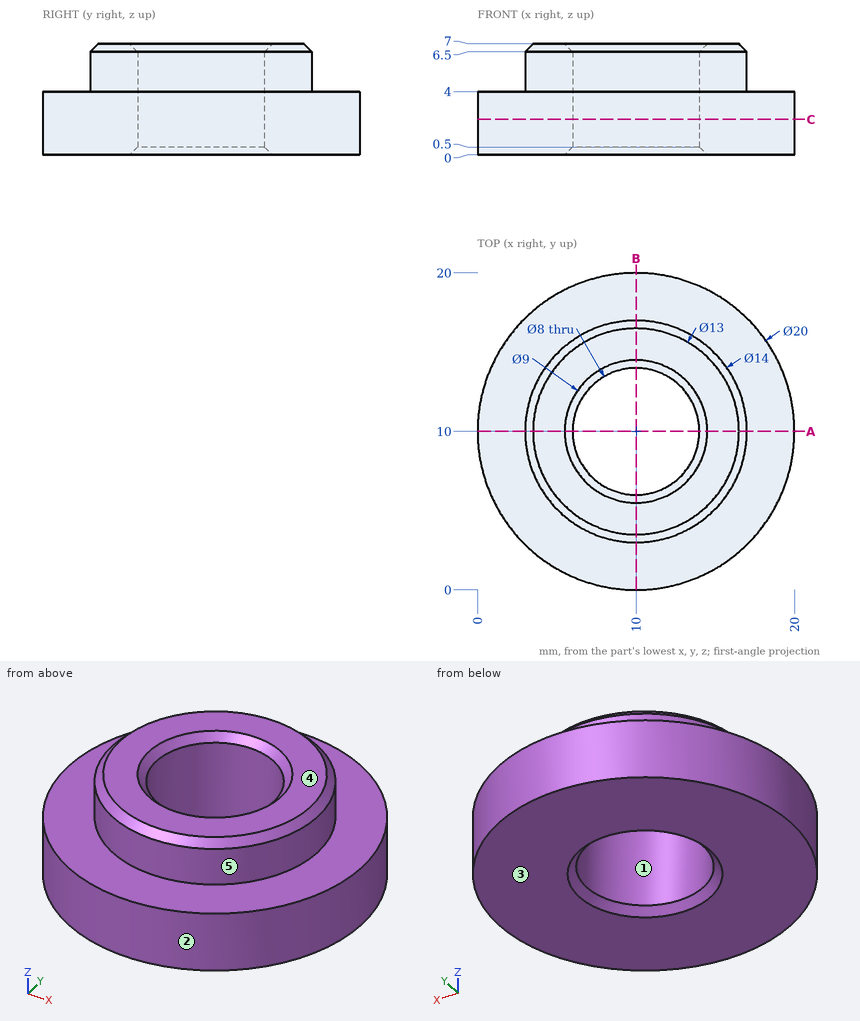
Input: dimensioned drawing with shaded views. Units: mm. Origin: part minimum x, y, z. A direction names the side the tool comes from. Coordinates: 2 decimals unless noted, no trailing zeros. Loops run counter-clockwise (first coordinate to the right, second up) from the corner with the lowest first, then second, coordinate; pieces in that order, holes last. Notation, with made-up numbers: M 17,-11.75 L 24,-11.75 A25 ccw 24,12.25 Z; hole C 0,33 d5. An arc over 180 degrees is marked long. One line per item, written item: value. Start each with the question number.
1) Draft query along Y for the marked faces 1, 2 and 3. Return one class per face: released by +Y, released by -Y, zero draft, split by the parting line, or undercut.
2) Material intervals for L1, parallel to Y at x = 10, z = 4.05; L2, parallel to Y at x = 10, z = 2.55; L3, parallel to Z at x = 2.25, y = 14.75, sorted ascending. Write a range as from..to.
3) Cut plane A-A (y = 10). Return loops of the section in (x, z), then the cut area to 4 significant figures.
4) Pin query (flat end, axial travel): P1, Ø2, axis at y = 17.5, z = 3.5, coming from the -X side; P2, Ø4, axis at x = 14, y = 8, coming from the -Z side; P3, Ø1, axis at x = 12.5, z = 4, coming from the -Y side; P4, Ø1.5, axis at x = 3, y = 18, coming from the +Z side. Return the tip coordinate at first contact, or that it passes through.
5) Reachability of the marked faces 4 and 5 from +Z, -Z, +X, -X, +Y, -Y: full face, straight path, thin tool, end or side. Return the list, or none.
6) Cut plane C-C (z = 2.25). Return loops of the section in (x, y).
Evaluation:
1. face 1: undercut
1. face 2: split by the parting line
1. face 3: zero draft
2. L1: 3..6, 14..17
2. L2: 0..6, 14..20
2. L3: 0..4
3. outline: M 0,0 L 5.5,0 L 6,0.5 L 6,6.5 L 5.5,7 L 3.5,7 L 3,6.5 L 3,4 L 0,4 Z; M 14,0.5 L 14.5,0 L 20,0 L 20,4 L 17,4 L 17,6.5 L 16.5,7 L 14.5,7 L 14,6.5 Z
3. area: 65.25 mm^2
4. P1: x = 2.4
4. P2: z = 0
4. P3: y = 0.2
4. P4: z = 4
5. face 4: +Z, +X, -X, +Y, -Y
5. face 5: +Z
6. outline: C 10,10 d20; hole C 10,10 d8
